Read the model definition and answer for the solid it produces. Units are mm, in the model's axes. Coordinates: 2 decimals unless noted, no trailing zeros. Loops run counter-clockwise (first coordinate to the right, second up) from the corner with the lowest first, then second, coordinate; pieces in that order, holes last.
from build123d import *

# Parameters (mm, degrees)
F0_R     = 29.464
F1_DEPTH = 2.3622
F2_R     = 1.524
F3_W     = 7.62
F3_H     = 24.003
F4_DEPTH = 0.0254
F5_R     = 1.524
F6_DEPTH = 0.508


with BuildPart() as f1:
    # F0 (on Top) → F1 (new body)
    with BuildSketch(Plane.XY):
        Circle(F0_R)
    extrude(amount=F1_DEPTH)

    # F2
    f2_edges = [f1.edges().sort_by_distance(p)[0] for p in [
        (-29.464, 0, 2.3622),
    ]]
    fillet(f2_edges, radius=F2_R)

    # F3 (on face) → F4 (cut)
    with BuildSketch(Plane.XY.offset(2.3622)):
        with Locations((-13.716, 0)):
            Rectangle(F3_W, F3_H)
        with Locations((-4.572, 0)):
            Rectangle(F3_W, F3_H)
        with Locations((4.572, 0)):
            Rectangle(F3_W, F3_H)
        with Locations((13.716, 0)):
            Rectangle(F3_W, F3_H)
    extrude(amount=-F4_DEPTH, mode=Mode.SUBTRACT)

    # F5 (on face) → F6 (join)
    with BuildSketch(Plane(origin=(0, 0, 0), x_dir=(1, 0, 0), z_dir=(0, 0, -1))):
        with Locations((-20.193, -12.7)):
            Circle(F5_R)
        with Locations((20.193, -12.7)):
            Circle(F5_R)
    extrude(amount=F6_DEPTH)


solid = f1.part
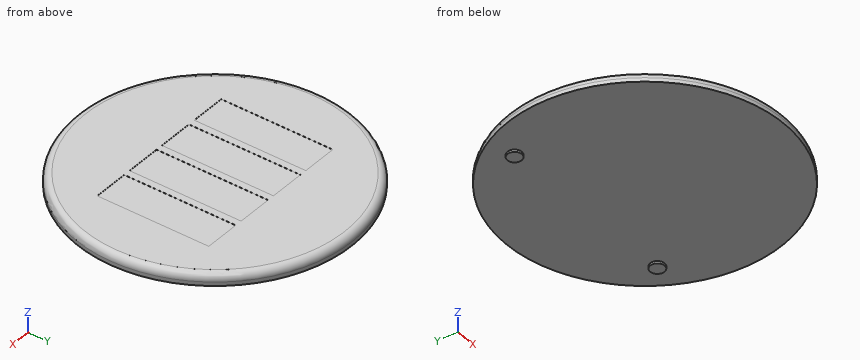
Item 1: Find the intervals of material crossed by line 1 along Z through (x, y) = (-9.5, -9); line 2 along Z through (x, y) = (-13.5, -10); line 3 along X through (y, z) = (-7.5, 0.35), in increasing order.
Numbers:
line 1: z = 0 to 2.36
line 2: z = 0 to 2.34
line 3: x = -28.49 to 28.49
Item 2: Given pin 1 (1 mm diameter, centred on y = -9, z = 0, fed in from -X); pin 2 (2 mm diameter, centred on x = 3, y = -15, fed in from -Z); pin 3 (1 mm diameter, centred on x = 19, z = 0.5, fed in from +Y), each flat-ended and moving along its own axis, determine where each tip first touches the part or whether it passes through.
Numbers:
pin 1: stops at x = -28.21
pin 2: stops at z = 0
pin 3: stops at y = 22.93
Item 3: A cutting plane is placed at C-C on z = 1.9. Determine the outline of the cut face in (x, y).
Numbers:
outline: circle Ø58.07 at (0, 0)
Item 4: A cutting plane is placed at B-B on x = 0. Determine the outline of the cut face in (y, z), then the cut area to 3 significant figures.
Numbers:
outline: (-29.46, 0) - (29.46, 0) - (29.46, 0.84) arc R1.52 ccw to (27.94, 2.36) - (-27.94, 2.36) arc R1.52 ccw to (-29.46, 0.84) - close
area: 138 mm2
